Work out the finished part from the listing and answer in its coordinate system (mm). A direction names the side the tool comes from. Round coordinates to 2 decimals unless told otherwise and drop trailing zeros. Loops run counter-clockwise (first coordinate to the right, second up) from the corner with the lowest first, then second, coordinate; pieces in that order, holes last.
```python
from build123d import *

# Parameters (mm, degrees)
SKETCH_1_W           = 75
SKETCH_1_H           = 100
EXTRUDE_1_DEPTH      = 3.6
CHAMFER_1_SIZE       = 10
SKETCH_2_W           = 5.2
SKETCH_2_H           = 15
SKETCH_2_W_2         = 15
SKETCH_2_H_2         = 13.5
EXTRUDE_2_DEPTH      = 30
SKETCH_3_W           = 15
SKETCH_3_H           = 30
EXTRUDE_3_DEPTH      = 2
SKETCH_4_W           = 13.5
SKETCH_4_H           = 30
EXTRUDE_4_DEPTH      = 12
SKETCH_5_R           = 2.2
CUT_EXTRUDE_1_DEPTH  = 115
SKETCH_6_W           = 49.4
SKETCH_6_H           = 18
EXTRUDE_5_DEPTH      = 25
SKETCH_8_R           = 1.665
CUT_EXTRUDE_3_DEPTH  = 25
EXTRUDE_7_REACH      = 71.327
SKETCH_10_R          = 1.6
CUT_EXTRUDE_4_DEPTH  = 130
SKETCH_12_R          = 1.6
CUT_EXTRUDE_6_DEPTH  = 120
CHAMFER_2_SIZE       = 10
SKETCH_15_W          = 3.6
SKETCH_15_H          = 13
CUT_EXTRUDE_8_DEPTH  = 23
SKETCH_16_R          = 4.155
CUT_EXTRUDE_9_DEPTH  = 4.5
SKETCH_17_W          = 13
SKETCH_17_H          = 23
CUT_EXTRUDE_10_DEPTH = 23
CUT_EXTRUDE_11_DEPTH = 33


with BuildPart() as part:
    # 草图1 → 凸台-拉伸1 (new body)
    with BuildSketch(Plane(origin=(0, 0, 0), x_dir=(1, 0, 0), z_dir=(0, 1, 0))):
        Rectangle(SKETCH_1_W, SKETCH_1_H)
    extrude(amount=EXTRUDE_1_DEPTH)

    # 倒角1
    chamfer_1_edges = [part.edges().sort_by_distance(p)[0] for p in [
        (37.5, 1.8, 50),
        (-37.5, 1.8, 50),
        (-37.5, 1.8, -50),
        (37.5, 1.8, -50),
    ]]
    chamfer(chamfer_1_edges, length=CHAMFER_1_SIZE)

    # 草图2 → 凸台-拉伸2 (add)
    with BuildSketch(Plane(origin=(0, 3.6, 0), x_dir=(1, 0, 0), z_dir=(0, 1, 0))):
        with Locations((-32.9, -10.5)):
            Rectangle(SKETCH_2_W, SKETCH_2_H)
        with Locations((18, -11.25)):
            Rectangle(SKETCH_2_W_2, SKETCH_2_H_2)
    extrude(amount=EXTRUDE_2_DEPTH)

    # 草图3 → 凸台-拉伸3 (add)
    with BuildSketch(Plane.ZY.offset(35.5)):
        with Locations((10.5, 18.6)):
            Rectangle(SKETCH_3_W, SKETCH_3_H)
    extrude(amount=EXTRUDE_3_DEPTH)

    # 草图4 → 凸台-拉伸4 (add)
    with BuildSketch(Plane(origin=(25.5, 0, 0), x_dir=(0, 0, -1), z_dir=(1, 0, 0))):
        with Locations((-11.25, 18.6)):
            Rectangle(SKETCH_4_W, SKETCH_4_H)
    extrude(amount=EXTRUDE_4_DEPTH)

    # 草图5 → 切除-拉伸1 (cut)
    with BuildSketch(Plane.XY.offset(18)):
        with Locations((-34.5, 21.6)):
            Circle(SKETCH_5_R)
        with Locations((-34.5, 11.6)):
            Circle(SKETCH_5_R)
        with Locations((15, 21.6)):
            Circle(SKETCH_5_R)
        with Locations((15, 11.6)):
            Circle(SKETCH_5_R)
    extrude(amount=-CUT_EXTRUDE_1_DEPTH, mode=Mode.SUBTRACT)

    # 草图6 → 凸台-拉伸5 (add)
    with BuildSketch(Plane(origin=(0, 3.6, 0), x_dir=(1, 0, 0), z_dir=(0, 1, 0))):
        with Locations((2.8, 33.2)):
            Rectangle(SKETCH_6_W, SKETCH_6_H)
    extrude(amount=EXTRUDE_5_DEPTH)

    # 草图8 → 切除-拉伸3 (cut)
    with BuildSketch(Plane.XY.offset(-24.2)):
        with Locations((0.65, 16.6)):
            Circle(SKETCH_8_R)
    extrude(amount=-CUT_EXTRUDE_3_DEPTH, mode=Mode.SUBTRACT)

    # 凸台-拉伸7: up to this face of the body (flat: up to its plane)
    extrude_7_end = Plane(part.part.faces().sort_by_distance((2.8, 28.6, -33.2))[0])
    # 草图9 → 凸台-拉伸7 (add, up to the picked face)
    with BuildSketch(Plane(origin=(0, 3.6, 0), x_dir=(1, 0, 0), z_dir=(0, 1, 0)), mode=Mode.PRIVATE) as extrude_7_sk1:
        Polygon((-21.9, 42.2), (-37.5, 42.2), (-37.5, -3), (-33.9, -3), (-33.9, 24.2), (-21.9, 24.2), align=None)
    extrude_7_tool1 = split(extrude(extrude_7_sk1.sketch, amount=EXTRUDE_7_REACH, mode=Mode.PRIVATE), bisect_by=extrude_7_end, keep=Keep.BOTH, mode=Mode.PRIVATE)
    # 草图9 → 凸台-拉伸7 (add, up to the picked face)
    with BuildSketch(Plane(origin=(0, 3.6, 0), x_dir=(1, 0, 0), z_dir=(0, 1, 0)), mode=Mode.PRIVATE) as extrude_7_sk2:
        Polygon((37.5, -4.5), (37.5, 42.2), (27.5, 42.2), (27.5, 24.2), (27.5, -4.5), align=None)
    extrude_7_tool2 = split(extrude(extrude_7_sk2.sketch, amount=EXTRUDE_7_REACH, mode=Mode.PRIVATE), bisect_by=extrude_7_end, keep=Keep.BOTH, mode=Mode.PRIVATE)
    add(extrude_7_tool1.solids().sort_by(Axis((-31.251331, 3.6, -27.356654), (0, 1, 0)))[0])
    add(extrude_7_tool2.solids().sort_by(Axis((32.5, 3.6, -18.85), (0, 1, 0)))[0])

    # 草图10 → 切除-拉伸4 (cut)
    with BuildSketch(Plane(origin=(0, 3.6, 0), x_dir=(1, 0, 0), z_dir=(0, 1, 0))):
        with Locations(Location((-7.5, 7.5, 0), (0, 0, 270))):
            Circle(SKETCH_10_R)
        with Locations(Location((7.5, 7.5, 0), (0, 0, 90))):
            Circle(SKETCH_10_R)
        with Locations(Location((7.5, -7.5, 0), (0, 0, 270))):
            Circle(SKETCH_10_R)
        with Locations(Location((-7.5, -7.5, 0), (0, 0, 90))):
            Circle(SKETCH_10_R)
    extrude(amount=-CUT_EXTRUDE_4_DEPTH, mode=Mode.SUBTRACT)

    # 草图12 → 切除-拉伸6 (cut)
    with BuildSketch(Plane(origin=(0, 3.6, 0), x_dir=(1, 0, 0), z_dir=(0, 1, 0))):
        with Locations(Location((-25.5, 45, 0), (0, 0, 270))):
            Circle(SKETCH_12_R)
        with Locations(Location((-10.5, 45, 0), (0, 0, 270))):
            Circle(SKETCH_12_R)
        with Locations(Location((10.5, 45, 0), (0, 0, 90))):
            Circle(SKETCH_12_R)
        with Locations(Location((25.5, 45, 0), (0, 0, 90))):
            Circle(SKETCH_12_R)
        with Locations(Location((25.5, -45, 0), (0, 0, 270))):
            Circle(SKETCH_12_R)
        with Locations(Location((10.5, -45, 0), (0, 0, 270))):
            Circle(SKETCH_12_R)
        with Locations(Location((-10.5, -45, 0), (0, 0, 90))):
            Circle(SKETCH_12_R)
        with Locations(Location((-25.5, -45, 0), (0, 0, 90))):
            Circle(SKETCH_12_R)
    extrude(amount=-CUT_EXTRUDE_6_DEPTH, mode=Mode.SUBTRACT)

    # 倒角2
    chamfer_2_edges = [part.edges().sort_by_distance(p)[0] for p in [
        (27.5, 16.1, -24.2),
        (-33.9, 16.1, -24.2),
    ]]
    chamfer(chamfer_2_edges, length=CHAMFER_2_SIZE)

    # 草图15 → 切除-拉伸8 (cut)
    with BuildSketch(Plane(origin=(0, 28.6, 0), x_dir=(1, 0, 0), z_dir=(0, 1, 0))):
        with Locations((-35.7, 3.5)):
            Rectangle(SKETCH_15_W, SKETCH_15_H)
    extrude(amount=-CUT_EXTRUDE_8_DEPTH, mode=Mode.SUBTRACT)

    # 草图16 → 切除-拉伸9 (cut)
    with BuildSketch(Plane.XY.offset(-24.2)):
        with Locations((0.65, 16.6)):
            Circle(SKETCH_16_R)
    extrude(amount=-CUT_EXTRUDE_9_DEPTH, mode=Mode.SUBTRACT)

    # 草图17 → 切除-拉伸10 (cut)
    with BuildSketch(Plane.ZY.offset(-27.5)):
        with Locations((-3.5, 17.1)):
            Rectangle(SKETCH_17_W, SKETCH_17_H)
    extrude(amount=-CUT_EXTRUDE_10_DEPTH, mode=Mode.SUBTRACT)

    # 草图18 → 切除-拉伸11 (cut)
    with BuildSketch(Plane.XZ):
        Polygon((-37.5, -40), (-35.3, -42.2), (-37.5, -42.2), align=None)
        Polygon((37.5, -42.2), (37.5, -40), (35.3, -42.2), align=None)
    extrude(amount=-CUT_EXTRUDE_11_DEPTH, mode=Mode.SUBTRACT)


solid = part.part
```
1. Find section A-A (x = -25.5). Write down the section's boundary in (y, z).
Answer key:
outline: (0, -50) - (3.6, -50) - (3.6, -46.6) - (0, -46.6) - close; (0, -43.4) - (3.6, -43.4) - (3.6, -42.2) - (28.6, -42.2) - (28.6, -22.6) - (3.6, -22.6) - (3.6, 43.4) - (0, 43.4) - close; (0, 46.6) - (3.6, 46.6) - (3.6, 50) - (0, 50) - close
2. Which of the six approach directions +Z, -Z, +X, -X, +Y, -Y give full straight-line access (tool end or side, diameter ignored) to faces 5 (the face through (-34, 33.6, 10)), 6 (the face through (2.567, 12.914, -26.418)), 7 (the face through (10.5, 18, 11)), 8 (the face through (0, 2, -50)), 9 (the face through (22.6, 15.9, -19.1))?
Answer key:
face 5: +Z, -Z, +X, -X, +Y
face 6: +Z
face 7: +Z, +Y
face 8: -Z, +X, -X, +Y, -Y
face 9: +Y
3. Determine the mould class of faces 1 (the face through (32.6, 1.8, 44.9)), 2 (the face through (-35.44, 11.06, -42.06)), 3 (the face through (-36.698, 11.697, 10.605)), 4 (the face through (-34, 18, 3)) for opening direction Z: +Z half, -Z half, draft (parallel to the pull), parting line (faces both ways), or undercut.
Answer key:
face 1: +Z half
face 2: -Z half
face 3: draft
face 4: undercut
4. Find section D-D (z = -19.5). Write down the section's boundary in (x, y).
Answer key:
outline: (-37.5, 0) - (37.5, 0) - (37.5, 28.6) - (22.2, 28.6) - (22.2, 3.6) - (-28.6, 3.6) - (-28.6, 28.6) - (-37.5, 28.6) - close
5. Find section B-B (y = 16.6). Give the number of separate pieces and of enclosed holes in the cut face, then the cut area to 3 significant figures.
Answer key:
separate pieces: 4
enclosed holes: 0
area: 2,040 mm2
6. Consider probe 1 along X at (y, z) = (0.8, 7.5); probe 2 along Y at (x, z) = (-33, 3.5); probe 3 along Y at (x, z) = (0.65, -27.5) (3 decimals). Determine where each line is inside the solid, lowest interval first.
Answer key:
probe 1: x = -37.5 to -9.1, -5.9 to 5.9, 9.1 to 37.5
probe 2: y = 0 to 9.99, 13.21 to 19.99, 23.21 to 33.6
probe 3: y = 0 to 12.445, 20.755 to 28.6
7. Given pin 1 (4 mm diameter, centred on x = -35, z = -2.5, fed in from +Y); pin 2 (10 mm diameter, centred on x = -17, z = 6, fed in from +Y); pin 3 (1 mm diameter, centred on x = -26.5, y = 9, fed in from +Z), each flat-ended and moving along its own axis, determine where each tip first touches the part or whether it passes through.
Answer key:
pin 1: stops at y = 5.6
pin 2: stops at y = 3.6
pin 3: stops at z = -21.1
8. Find section C-C (y = 26.5). Write down the section's boundary in (x, z).
Answer key:
outline: (-37.5, -40) - (-35.3, -42.2) - (35.3, -42.2) - (37.5, -40) - (37.5, -10) - (27.5, -10) - (27.5, -14.2) - (17.5, -24.2) - (-23.9, -24.2) - (-33.9, -14.2) - (-33.9, -10) - (-37.5, -10) - close; (-37.5, 3) - (-30.3, 3) - (-30.3, 18) - (-37.5, 18) - close; (10.5, 4.5) - (27.5, 4.5) - (27.5, 3) - (37.5, 3) - (37.5, 18) - (10.5, 18) - close
